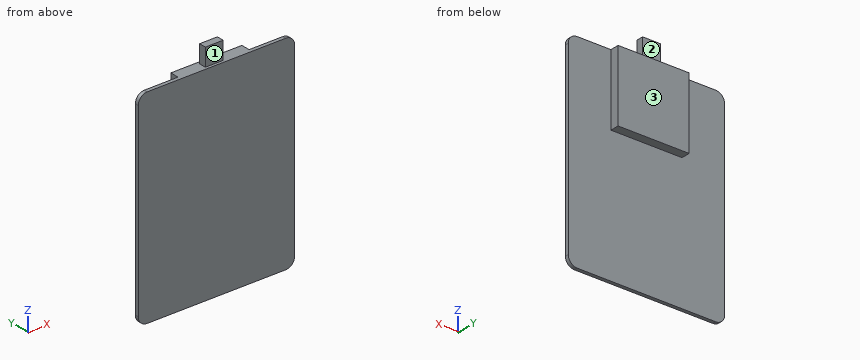
```python
from build123d import *

# Parameters (mm, degrees)
BOSS_EXTRUDE4_DEPTH = 2
SKETCH6_W           = 40
SKETCH6_H           = 40
BOSS_EXTRUDE5_DEPTH = 5
SKETCH7_W           = 10
SKETCH7_H           = 4
BOSS_EXTRUDE6_DEPTH = 10


with BuildPart() as part:
    # Sketch5 → Boss-Extrude4 (new body)
    with BuildSketch(Plane(origin=(0, 0, 0), x_dir=(1, 0, 0), z_dir=(0, 1, 0))):
        with BuildLine():
            Line((39, 57.5), (-39, 57.5))
            ThreePointArc((-39, 57.5), (-42.535533906, 56.035533906), (-44, 52.5))
            Line((-44, 52.5), (-44, -52.5))
            ThreePointArc((-44, -52.5), (-42.535533906, -56.035533906), (-39, -57.5))
            Line((-39, -57.5), (39, -57.5))
            ThreePointArc((39, -57.5), (42.535533906, -56.035533906), (44, -52.5))
            Line((44, -52.5), (44, 52.5))
            ThreePointArc((44, 52.5), (42.535533906, 56.035533906), (39, 57.5))
        make_face()
    extrude(amount=BOSS_EXTRUDE4_DEPTH)

    # Sketch6 → Boss-Extrude5 (add)
    with BuildSketch(Plane(origin=(0, 2, 0), x_dir=(1, 0, 0), z_dir=(0, 1, 0))):
        with Locations((0, -37.5)):
            Rectangle(SKETCH6_W, SKETCH6_H)
    extrude(amount=BOSS_EXTRUDE5_DEPTH)

    # Sketch7 → Boss-Extrude6 (add)
    with BuildSketch(Plane.XY.offset(57.5)):
        with Locations((0, 3.5)):
            Rectangle(SKETCH7_W, SKETCH7_H)
    extrude(amount=BOSS_EXTRUDE6_DEPTH)


solid = part.part
```
Source: CAD feature listing. Evaluate the final solid. Frame: model axes, mm. Face numbers are marked on the shaded views. A direction names the side the tool comes from. Round coordinates to 2 decimals unless told otherwise and drop trailing zeros. Loops run counter-clockwise (first coordinate to the right, second up) from the corner with the lowest first, then second, coordinate; pieces in that order, holes last.
(1) Section query D-D (z = -17.5). Output: boundary loops of the cut face in (x, y), and give its area (3 significant figures).
From the geometry:
outline: (-44, 0) - (44, 0) - (44, 2) - (-44, 2) - close
area: 176 mm2
(2) Contact query for flat-ended pins moving along their axis: pin 1 Ø2.5 at (x, y) = (2, 5.5) entering from -Z; pin 2 Ø1 at (x, y) = (17, 2.5) entering from +Z; pin 3 Ø3 at (y, z) = (5, 34) entering from -X; pin 4 Ø2 at (x, y) = (29, 4.5) entering from +Z. Output: stop coordinate, or through.
From the geometry:
pin 1: stops at z = 17.5
pin 2: stops at z = 57.5
pin 3: stops at x = -20
pin 4: passes through
(3) Access query for the marked faces 1, 2 and 3. Directions: +Z, -Z, +X, -X, +Y, -Y. A direction counts if a zero-diameter tool reaches every point of the face in a straight line with its end or side. Return the directions, or none.
From the geometry:
face 1: +Z, +X, -X, -Y
face 2: +Z, +X, -X, +Y
face 3: +Z, -Z, +X, -X, +Y
(4) Section query C-C (x = 2). Output: boundary loops of the cut face in (y, z), and give its area (3 significant figures).
From the geometry:
outline: (0, -57.5) - (2, -57.5) - (2, 17.5) - (7, 17.5) - (7, 57.5) - (5.5, 57.5) - (5.5, 67.5) - (1.5, 67.5) - (1.5, 57.5) - (0, 57.5) - close
area: 470 mm2
(5) Section query B-B (z = 47.5). Output: boundary loops of the cut face in (x, y).
From the geometry:
outline: (-44, 0) - (44, 0) - (44, 2) - (20, 2) - (20, 7) - (-20, 7) - (-20, 2) - (-44, 2) - close
(6) Section query A-A (y = 4.25). Output: boundary loops of the cut face in (x, z), and give its area (3 significant figures).
From the geometry:
outline: (-20, 17.5) - (20, 17.5) - (20, 57.5) - (5, 57.5) - (5, 67.5) - (-5, 67.5) - (-5, 57.5) - (-20, 57.5) - close
area: 1,700 mm2
(7) Material intervals for probe 1 along X at (y, z) = (4.5, 38); probe 2 along Z at (x, y) = (-3.5, 4.75); probe 3 along X at (y, z) = (5.25, 59), sorted ascending.
From the geometry:
probe 1: x = -20 to 20
probe 2: z = 17.5 to 67.5
probe 3: x = -5 to 5
